Verification items for the finished model (mm, model axes). A direction names the side the tool comes from. Coordinates: 2 decimals unless noted, no trailing zeros. Loops run counter-clockwise (first coordinate to the right, second up) from the corner with the lowest first, then second, coordinate; pieces in that order, holes last.
Q1. Go/stop test with flat-tipped pins: P1, Ø2.5, axis at x = 0, z = 47, coming from the +Y side; P2, Ø3, axis at x = -33.5, y = 0.5, coming from the -Z side; P3, Ø1.2, axis at x = -31.5, y = 2.5, coming from the +Z side; P4, Ø4.5, axis at y = 1.5, z = -0.5, coming from the +X side. Record where each tip stops, or that it passes through.
Q2. Sectioned sample at C-C (y = -1.5). Enter the section's corners in (x, z).
Q3. Material ranges on probe 1 along Z at (x, y) = (0, 2); probe 2 along X at (y, z) = (9.5, -43.5); probe 3 along X at (y, z) = (6.75, -48), recorded low to high.
Q4. Sectioned sample at A-A (y = 8.25). Count the separate pieces of the cut face and the enclosed holes in it, then the cut area to 3 significant figures.
Q5. Mould release check, pull along Z, two halves, no side actions. Record for faces 1 (the face through (-0.8, -6.6, -11.5)), 2 (the face through (26.76, 3.3, -51.46)), 3 (the face through (43, 10, -2)): +Z half, -Z half, draft (parallel to the pull), parting line (faces both ways), or undercut.
Q6. Access from +Z, -Z, +X, -X, +Y, -Y to the whole of each face (thin tool, end or side, straight path). Record for faces 4 (the face through (0.1, -3.3, -11.1)), 5 (the face through (0, 0, -47)).
Autodesk Inventor part; units mm, degrees
ref_plane "YZ Plane" through (0, 0, 0) normal (1, 0, 0) x (0, 1, 0)
ref_plane "XZ Plane" through (0, 0, 0) normal (0, 1, 0) x (-1, 0, 0)
ref_plane "XY Plane" through (0, 0, 0) normal (0, 0, 1) x (1, 0, 0)
sketch "Sketch1" plane through (0, 0, 0) normal (0, 1, 0) x (-1, 0, 0)
  circle A0 centre (0, 0) radius 55
  dimension "d4" = 110
sketch "Sketch2" plane through (0, 0, 0) normal (0, 1, 0) x (-1, 0, 0)
  circle A0 centre (0, 0) radius 40 construction
  circle A1 centre (0, 0) radius 47.5 construction
  circle A2 centre (0, 47.5) radius 4.5
  circle A3 centre (0, 47.5) radius 6.5
  dimension "d11" = 95
  dimension "d10" = 80
  dimension "d12" = 9
  dimension "d13" = 13
extrude "Extrusion1" add sketch "Sketch1" against normal blind 6.6
extrude "Extrusion2" add sketch "Sketch2" along normal blind 10
pattern_circular "Circular Pattern1" count 4 over 360 about axis through (0, -10, 0) along (0, 1, 0) of "Extrusion2"
sketch "Sketch3" plane through (0, -6.6, 0) normal (0, -1, 0) x (1, 0, 0)
  circle A0 centre (0, 0) radius 55
  circle A1 centre (0, 0) radius 55
  circle A2 centre (0, 0) radius 58
  dimension "d21" = 116
extrude "Extrusion3" add sketch "Sketch3" against normal blind 17
sketch "Sketch4" plane through (0, 0, 0) normal (0, 1, 0) x (1, 0, 0)
  circle A0 centre (0, 0) radius 8.1
  dimension "d24" = 16.2
extrude "Extrusion4" cut sketch "Sketch4" against normal blind 30
sketch "Sketch6" plane through (0, 0, 0) normal (1, 0, 0) x (0, 1, 0)
  line L0 (0, 8.1) -> (0, -8.1)
  line L1 (-6.6, -58) -> (-6.6, 58)
  line L2 (0, 8.1) -> (-6.6, 8.1)
  line L3 (-6.6, 8.1) -> (-6.6, 11.1)
  line L4 (-6.6, 11.1) -> (0, 11.1)
  line L5 (0, 11.1) -> (0, 8.1)
  line L6 (-8.4, 0) -> (1.4, 0)
  point P0 (0, 0)
  dimension "d27" = 3
revolve "Revolution1" cut sketch "Sketch6" angle 40 mid plane about axis through (0, -10, 0) along (0, 1, 0) contours L2 L1 L4 L5
pattern_circular "Circular Pattern2" count 4 over 360 about axis through (0, -10, 0) along (0, 1, 0) of "Revolution1"
fillet "Fillet1" radius 3 1 edges at (-58, -6.6, 0)
sketch "Sketch7" plane through (0, 0, 0) normal (0, 1, 0) x (1, 0, 0)
  circle A0 centre (0, 0) radius 12.5 construction
  line L0 (-12.144, 5.5) -> (-39.644, 5.5)
  line L1 (-39.644, 5.5) -> (-39.644, -5.5)
  line L2 (-39.644, -5.5) -> (-12.144, -5.5)
  line L3 (-12.144, -5.5) -> (-12.144, 5.5)
  dimension "d33" = 25
  dimension "d34" = 27.5
  dimension "d35" = 11
  dimension "d36" = 5.5
extrude "Extrusion5" add sketch "Sketch7" along normal blind 4
properties part number "BaseHumedadDireccion"
Geometry check:
1. P1: stops at y = 0
1. P2: stops at z = -48.37
1. P3: stops at z = 49.08
1. P4: stops at x = 58
2. outline: circle Ø116 at (0, 0); hole (-10.43, -3.8) - (-7.61, -2.77) arc R8.1 ccw to (-2.77, -7.61) - (-3.8, -10.43) arc R11.1 ccw to (3.8, -10.43) - (2.77, -7.61) arc R8.1 ccw to (7.61, -2.77) - (10.43, -3.8) arc R11.1 ccw to (10.43, 3.8) - (7.61, 2.77) arc R8.1 ccw to (2.77, 7.61) - (3.8, 10.43) arc R11.1 ccw to (-3.8, 10.43) - (-2.77, 7.61) arc R8.1 ccw to (-7.61, 2.77) - (-10.43, 3.8) arc R11.1 ccw to start
3. probe 1: z = -58 to -55, -54 to -52, -43 to -41, 41 to 43, 52 to 54, 55 to 58
3. probe 2: x = -38.36 to -33.66, -5.12 to -2.06, 2.06 to 5.12, 33.66 to 38.36
3. probe 3: x = -32.56 to -26.85, -6.48 to -4.47, 4.47 to 6.48, 26.85 to 32.56
4. separate pieces: 5
4. enclosed holes: 5
4. area: 1,340 mm2
5. face 1: draft
5. face 2: parting line
5. face 3: undercut
6. face 4: +Y, -Y
6. face 5: +Y
